The drawing under review shows one solid part. Ordinate dimensions are in mm from its lowest x, y, z. Round coordinates to 2 decimals unless told otherwise and drop trailing zeros. Order: outer loops, then holes, each group sorted by start corner. A loop starts at its lowest first (then second) coordinate and runs counter-clockwise, first axis right, second up. Notation, with made-up numbers: M 70.5,36 L 124.5,36 A25 cw 124.5,74 Z; hole C 15,7.25 d10. An arc over 180 degrees is marked long. Use a Markdown table: item, result.
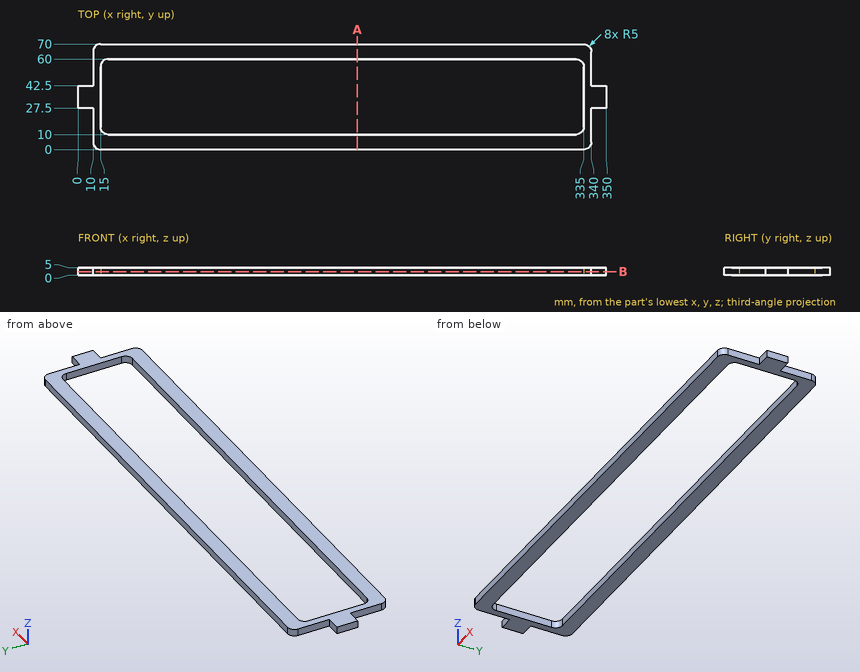
Q1. Add section A-A (x = 185). Write out the cut boundary in (y, z), then the cut area to 3 significant figures.
Determined:
| item | result |
|---|---|
| outline | M 0,0 L 10,0 L 10,5 L 0,5 Z; M 60,0 L 70,0 L 70,5 L 60,5 Z |
| area | 100 mm^2 |
Q2. Clearance check with flat-ended pins moving along their axes: pin 1 (1.5 mm diameter, centred on y = 58.5, z = 2.5, fed in from -X); pin 2 (1.5 mm diameter, centred on y = 37.5, z = 2, fed in from -X); pin 3 (1.5 mm diameter, centred on y = 54, z = 3, fed in from +X); pin 4 (2.5 mm diameter, centred on x = 342.5, z = 2.5, fed in from -Y). State where each tip first meets the part, or that it passes through.
Determined:
| item | result |
|---|---|
| pin 1 | stops at x = 10 |
| pin 2 | stops at x = 0 |
| pin 3 | stops at x = 340 |
| pin 4 | stops at y = 27.5 |
Q3. Wall thickness on line 1 along Y through (x, z) = (132, 1.7); line 2 along X through (y, z) = (54.5, 0.85); line 3 along X through (y, z) = (39, 1.9): over which ranges is each line inside the solid? List them lowest first. Write a range as [from, to].
Determined:
| item | result |
|---|---|
| line 1 | y = [0, 10], [60, 70] |
| line 2 | x = [10, 15], [335, 340] |
| line 3 | x = [0, 15], [335, 350] |
Q4. Add section B-B (z = 2.4). Write out the cut boundary in (x, y).
Determined:
| item | result |
|---|---|
| outline | M 0,27.5 L 10,27.5 L 10,5 A5 ccw 15,0 L 335,0 A5 ccw 340,5 L 340,27.5 L 350,27.5 L 350,42.5 L 340,42.5 L 340,65 A5 ccw 335,70 L 15,70 A5 ccw 10,65 L 10,42.5 L 0,42.5 Z; hole M 15,15 A5 ccw 20,10 L 330,10 A5 ccw 335,15 L 335,55 A5 ccw 330,60 L 20,60 A5 ccw 15,55 Z |
